Can you work these out from the model? Positions are in its coordinate system, mm. Face numbers are marked on the shaded views. A direction names the side the tool comes from. Round coordinates to 2 decimals unless told otherwise and drop trailing zeros. Loops run counter-clockwise (first coordinate to the right, second up) from the corner with the lowest first, then second, coordinate; pieces in that order, holes last.
```python
from build123d import *

# Parameters (mm, degrees)
F0_W      = 25
F0_H      = 12
F1_DEPTH  = 12
F2_R      = 8.05
F3_DEPTH  = 6.6
F4_R      = 6.05
F5_DEPTH  = 5.4
F6_W      = 12
F6_H      = 12
F7_DEPTH  = 3
F8_W      = 12
F8_H      = 12
F9_DEPTH  = 3
F10_R     = 1.25
F11_DEPTH = 25
F12_SIZE  = 1.5
F13_R     = 0.99999
F14_W     = 10
F14_H     = 2
F15_DEPTH = 5
F16_W     = 10
F16_H     = 2
F17_DEPTH = 5
F19_DEPTH = 2
F20_R     = 3


# Not quite as in the source:
# - a fillet or chamfer is up to 0.001 mm smaller than in the source, because OpenCascade refuses the exact size


with BuildPart() as f1:
    # F0 (on Top) → F1 (new body)
    with BuildSketch(Plane.XY):
        with Locations((12.5, 6)):
            Rectangle(F0_W, F0_H)
    extrude(amount=F1_DEPTH)

    # F2 (on face) → F3 (cut)
    with BuildSketch(Plane.XZ):
        with Locations((12.5, 12)):
            Circle(F2_R)
    extrude(amount=-F3_DEPTH, mode=Mode.SUBTRACT)

    # F4 (on face) → F5 (cut)
    with BuildSketch(Plane(origin=(0, 12, 0), x_dir=(-1, 0, 0), z_dir=(0, 1, 0))):
        with Locations((-12.5, 12)):
            Circle(F4_R)
    extrude(amount=-F5_DEPTH, mode=Mode.SUBTRACT)

    # F6 (on face) → F7 (join)
    with BuildSketch(Plane(origin=(0, 0, 0), x_dir=(0, -1, 0), z_dir=(-1, 0, 0))):
        with Locations((-6, 6)):
            Rectangle(F6_W, F6_H)
    extrude(amount=F7_DEPTH)

    # F8 (on face) → F9 (join)
    with BuildSketch(Plane.YZ.offset(25)):
        with Locations((6, 6)):
            Rectangle(F8_W, F8_H)
    extrude(amount=F9_DEPTH)

    # F10 (on face) → F11 (cut)
    with BuildSketch(Plane.XY.offset(12)):
        with Locations((0.75, 7.55)):
            Circle(F10_R)
        with Locations((24.25, 7.55)):
            Circle(F10_R)
    extrude(amount=-F11_DEPTH, mode=Mode.SUBTRACT)

    # F12
    f12_edges = [f1.edges().sort_by_distance(p)[0] for p in [
        (23, 7.55, 0),
        (-0.5, 7.55, 0),
    ]]
    chamfer(f12_edges, length=F12_SIZE)

    # F13 (radius 1 in the source; OpenCascade refuses exactly that, so slightly less here)
    f13_edges = [f1.edges().sort_by_distance(p)[0] for p in [
        (28, 6, 0),
        (-3, 6, 0),
        (28, 12, 6),
        (12.5, 12, 0),
        (-3, 12, 6),
        (-3, 0, 6),
        (12.5, 0, 0),
        (28, 0, 6),
    ]]
    fillet(f13_edges, radius=F13_R)

    # F14 (on face) → F15 (join)
    with BuildSketch(Plane.YZ.offset(28)):
        with Locations((6, 11)):
            Rectangle(F14_W, F14_H)
    extrude(amount=F15_DEPTH)

    # F16 (on face) → F17 (join)
    with BuildSketch(Plane(origin=(-3, 0, 0), x_dir=(0, -1, 0), z_dir=(-1, 0, 0))):
        with Locations((-6, 11)):
            Rectangle(F16_W, F16_H)
    extrude(amount=F17_DEPTH)

    # F18 (on face) → F19 (cut, through all)
    with BuildSketch(Plane.XY.offset(12)):
        with BuildLine():
            ThreePointArc((-4.25, 7.5), (-5.5, 8.75), (-6.75, 7.5))
            Line((-6.75, 7.5), (-6.75, 4.5))
            ThreePointArc((-6.75, 4.5), (-5.5, 3.25), (-4.25, 4.5))
            Line((-4.25, 4.5), (-4.25, 7.5))
        make_face()
        with BuildLine():
            ThreePointArc((31.75, 7.5), (30.5, 8.75), (29.25, 7.5))
            Line((29.25, 7.5), (29.25, 4.5))
            ThreePointArc((29.25, 4.5), (30.5, 3.25), (31.75, 4.5))
            Line((31.75, 4.5), (31.75, 7.5))
        make_face()
    extrude(amount=-F19_DEPTH, mode=Mode.SUBTRACT)

    # F20
    f20_edges = [f1.edges().sort_by_distance(p)[0] for p in [
        (-8, 11, 11),
        (-8, 1, 11),
        (33, 11, 11),
        (33, 1, 11),
    ]]
    fillet(f20_edges, radius=F20_R)


solid = f1.part
```
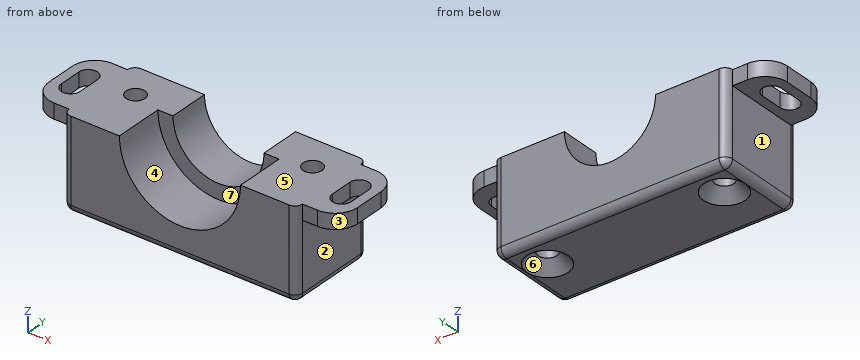
(1) We'd pull the mould along Y, two halves only. Please class the marked faces 5, 6 and 7: released by +Y, released by -Y, zero draft, split by the parting line, or undercut.
(2) For pin 1 (6 mm diameter, centred on y = 3.5, z = 5, fed in from -X); pin 2 (4 mm diameter, centred on x = 29.5, y = 6, fed in from -Z); pin 3 (3 mm diameter, centred on x = 0.75, y = 7.55, fed in from -Z); pin 4 (4 mm diameter, centred on x = 6, z = 9.5, fed in from -Y), each with a flat end and sliding along its axis, tell me the tip position at first contact or that it passes through.
(3) If I drill on line 1 (X direction, y = 7.5, z = 3.25); line 2 (Y direction, x = 0.75, z = 9.75); line 3 (X direction, y = 8.25, z = 2), over which ranges is the centre line in solid material (lowest first)?
(4) Suppose I cut it at D-D (x = -5.5). Write out the boundary of the cut face in (y, z).
(5) Suppose I cut it at C-C (z = 9.25). Write out the boundary of the cut face in (x, y), then the cut area to 3 significant figures.
(6) Suppose I cut it at B-B (z = 3.25). Write out the boundary of the cut face in (x, y), then the cut area to 3 significant figures.
(7) Which directions (+Z, -Z, +X, -X, +Y, -Y) give clear straight access to the entire face, cutting with the end or side of a thin tool? Please do the marked faces 1, 2, 3 and 4.
(8) Suppose I cut it at A-A (x = 0.75). Write out the boundary of the cut face in (y, z).
Check result:
1. face 5: zero draft
1. face 6: undercut
1. face 7: released by -Y
2. pin 1: stops at x = -3
2. pin 2: stops at z = 0.13
2. pin 3: stops at z = 1.25
2. pin 4: stops at y = 0
3. line 1: x = -3 to -0.5, 2 to 23, 25.5 to 28
3. line 2: y = 0 to 6.3, 8.8 to 12
3. line 3: x = -3 to -0.29, 1.79 to 23.21, 25.29 to 28
4. outline: (1.04, 10) - (3.25, 10) - (3.25, 12) - (1.04, 12) - close; (8.75, 10) - (10.96, 10) - (10.96, 12) - (8.75, 12) - close
5. outline: (-3, 1) arc R1 ccw to (-2, 0) - (4.93, 0) - (4.93, 6.6) - (7.11, 6.6) - (7.11, 12) - (-2, 12) arc R1 ccw to (-3, 11) - close; (17.89, 6.6) - (20.07, 6.6) - (20.07, 0) - (27, 0) arc R1 ccw to (28, 1) - (28, 11) arc R1 ccw to (27, 12) - (17.89, 12) - close; hole circle Ø2.5 at (0.75, 7.55); hole circle Ø2.5 at (24.25, 7.55)
5. area: 203 mm2
6. outline: (-3, 1) arc R1 ccw to (-2, 0) - (27, 0) arc R1 ccw to (28, 1) - (28, 11) arc R1 ccw to (27, 12) - (-2, 12) arc R1 ccw to (-3, 11) - close; hole circle Ø2.5 at (0.75, 7.55); hole circle Ø2.5 at (24.25, 7.55)
6. area: 361 mm2
7. face 1: -Z, -X, +Y, -Y
7. face 2: -Z, +X, +Y, -Y
7. face 3: +Z, -Z, +X, -Y
7. face 4: +Z, -Y
8. outline: (0, 1) arc R1 ccw to (1, 0) - (4.8, 0) - (6.3, 1.5) - (6.3, 12) - (0, 12) - close; (8.8, 1.5) - (10.3, 0) - (11, 0) arc R1 ccw to (12, 1) - (12, 12) - (8.8, 12) - close
